```python
from build123d import *

# Parameters (mm, degrees)
SKETCH1_RX          = 4
SKETCH1_RY          = 3
BOSS_EXTRUDE1_DEPTH = 4
BOSS_EXTRUDE1_TAPER = -33
SKETCH2_R           = 2
CUT_EXTRUDE1_DEPTH  = 10


with BuildPart() as part:
    # Sketch1 → Boss-Extrude1 (new body)
    with BuildSketch(Plane(origin=(0, 0, 0), x_dir=(1, 0, 0), z_dir=(0, 1, 0))):
        with Locations(Location((0, 0), (0, 0, 90))):
            Ellipse(SKETCH1_RX, SKETCH1_RY)
    extrude(amount=BOSS_EXTRUDE1_DEPTH, taper=BOSS_EXTRUDE1_TAPER)

    # Sketch2 → Cut-Extrude1 (cut)
    with BuildSketch(Plane.XZ):
        with Locations(Location((0, 0, 0), (0, 0, 270))):
            Circle(SKETCH2_R)
    extrude(amount=-CUT_EXTRUDE1_DEPTH, mode=Mode.SUBTRACT)


solid = part.part
```
The model under review builds one solid part; all positions refer to its coordinate system, in mm. Give positions to 0.01 mm unless a question says otherwise; leave off trailing zeros. Put each result on its own line as item: value.
(1) For pin 1 Ø2.5 at (x, z) = (0, 0) entering from +Y; pin 2 Ø1 at (y, z) = (0.5, 3.5) entering from -X; pin 3 Ø1 at (x, y) = (-0.5, 3) entering from -Z; pin 4 Ø1 at (x, y) = (0.5, 1) entering from -Z, all flat-tipped, find the tip position at first contact; note any pin that passes through.
Results are:
pin 1: through
pin 2: x = -2.58
pin 3: z = -6.25
pin 4: z = -4.94
(2) To check wall thickness, follow probe 1 along X at (y, z) = (2.1, 0); probe 2 along Z at (x, y) = (0.5, 1.2); probe 3 along X at (y, z) = (1.7, 0). State the ranges of each line that lie inside material, in increasing order. Write a range as from..to.
Results are:
probe 1: -4.36..-2, 2..4.36
probe 2: -4.74..-1.94, 1.94..4.74
probe 3: -4.1..-2, 2..4.1
(3) The part is to be moulded in two halves that separate along X. For faces 1 (the flat face through (1, 0, -2)), 2 (the cylindrical face through (-2, 2, 0)), say which applies: pulls with the +X half, pulls with the -X half, needs draft (parallel to the pull), parting line crosses it, or undercut.
Results are:
face 1: needs draft
face 2: undercut
